The listing builds one solid part. Answer for the finished solid, in the listing's coordinates (mm). Round coordinates to 2 decimals unless told otherwise and drop trailing zeros. Loops run counter-clockwise (first coordinate to the right, second up) from the corner with the lowest first, then second, coordinate; pieces in that order, holes last. Notation, with made-up numbers: M 2.5,41 L 53.5,41 A25 ccw 53.5,62 Z; hole C 89,65 d3. An arc over 180 degrees is marked long. Put each result on its own line as item: value. Start each with the question number.
(1) Flat-ended cylindrical pins translate along their axes: P1, Ø2, axis at x = 22, y = 10.5, coming from the +Z side; P2, Ø1.5, axis at y = 6, z = -8.5, coming from the -X side; P3, Ø1, axis at x = -13.5, y = 4, coming from the -Z side. Find the tip coordinate at first contact, or state that the pin passes through.
(2) Section B-B, the plane z = 11 is taken. Determine the outline of the cut face in (x, y).
(3) Section C-C, the plane x = 1 is taken. Determine the outline of the cut face in (y, z), then the cut area to 3 significant figures.
(4) Determine the mould class of faces 1 (the face through (-21.5, 8.38, 12.26)), 2 (the face through (-14.71, 8.38, 25.28)), 3 (the face through (-14.54, 8.38, -25.38)) for opening direction Z: released by +Z, released by -Z, zero draft, split by the parting line, or undercut.
(5) Straight lines are drawn through the part: line 1 (X direction, y = 13.25, z = 14.5); line 2 (X direction, y = 5.75, z = 18.5); line 3 (Z direction, x = -17.5, y = 13.5). For each, find the intervals that lie inside material, in ascending order.
(6) Section A-A, the plane y = 5 is taken. Determine the outline of the cut face in (x, z), then the cut area to 3 significant figures.
```python
from build123d import *

# Parameters (mm, degrees)
SALIENTE_EXTRUIR1_DEPTH = 17


with BuildPart() as part:
    # Croquis1 → Saliente-Extruir1 (new body)
    with BuildSketch(Plane(origin=(0, 0, 0), x_dir=(1, 0, 0), z_dir=(0, 1, 0))):
        with BuildLine():
            ThreePointArc((8.25, -28.062430401), (14.625, -25.331243061), (20.177777619, -21.175924782))
            ThreePointArc((20.177777619, -21.175924782), (21.434128744, -12.375), (28.427777619, -6.886505619))
            ThreePointArc((28.427777619, -6.886505619), (29.25, 0), (28.427777619, 6.886505619))
            ThreePointArc((28.427777619, 6.886505619), (21.434128744, 12.375), (20.177777619, 21.175924782))
            ThreePointArc((20.177777619, 21.175924782), (14.625, 25.331243061), (8.25, 28.062430401))
            ThreePointArc((8.25, 28.062430401), (0, 24.75), (-8.25, 28.062430401))
            ThreePointArc((-8.25, 28.062430401), (-14.625, 25.331243061), (-20.177777619, 21.175924782))
            ThreePointArc((-20.177777619, 21.175924782), (-21.434128744, 12.375), (-28.427777619, 6.886505619))
            ThreePointArc((-28.427777619, 6.886505619), (-29.25, 0), (-28.427777619, -6.886505619))
            ThreePointArc((-28.427777619, -6.886505619), (-21.434128744, -12.375), (-20.177777619, -21.175924782))
            ThreePointArc((-20.177777619, -21.175924782), (-14.625, -25.331243061), (-8.25, -28.062430401))
            ThreePointArc((-8.25, -28.062430401), (0, -24.75), (8.25, -28.062430401))
        make_face()
    extrude(amount=SALIENTE_EXTRUIR1_DEPTH)


solid = part.part
```
Recorded:
1. P1: stops at z = 13.2
1. P2: stops at x = -26.27
1. P3: stops at z = -26.2
2. outline: M -22.36,0 L 22.36,0 L 22.36,17 L -22.36,17 Z
3. outline: M 0,-24.79 L 17,-24.79 L 17,24.79 L 0,24.79 Z
3. area: 843 mm²
4. face 1: undercut
4. face 2: released by +Z
4. face 3: released by -Z
5. line 1: x = -20.47 to 20.47
5. line 2: x = -19.84 to 19.84
5. line 3: z = -23.44 to 23.44
6. outline: M -28.43,-6.89 A11.93 cw -20.18,-21.18 A29.25 ccw -8.25,-28.06 A11.93 cw 8.25,-28.06 A29.25 ccw 20.18,-21.18 A11.93 cw 28.43,-6.89 A29.25 ccw 28.43,6.89 A11.93 cw 20.18,21.18 A29.25 ccw 8.25,28.06 A11.93 cw -8.25,28.06 A29.25 ccw -20.18,21.18 A11.93 cw -28.43,6.89 A29.25 ccw Z
6. area: 2,380 mm²
